Autodesk Inventor part; units mm, degrees
ref_plane "YZ Plane" through (0, 0, 0) normal (1, 0, 0) x (0, 1, 0)
ref_plane "XZ Plane" through (0, 0, 0) normal (0, 1, 0) x (-1, 0, 0)
ref_plane "XY Plane" through (0, 0, 0) normal (0, 0, 1) x (1, 0, 0)
sketch "Sketch1" plane through (0, 0, 0) normal (0, 0, 1) x (1, 0, 0)
  line L0 (-50.8, -25.4) -> (76.2, -25.4)
  line L1 (76.2, -25.4) -> (76.2, 228.6)
  line L2 (76.2, 228.6) -> (-51.6296, 228.6)
  circle A0 centre (5.08, -4.9022) radius 1.905
  circle A1 centre (-1.27, 63.6778) radius 3.175
  circle A2 centre (13.97, 89.0778) radius 3.175
  arc A3 (23.4649, 83.1687) -> (9.3315, 59.465) centre (29.21, 63.6778) ccw
  arc A4 (0.3002, -6.6225) -> (5.08, -9.9822) centre (5.08, -4.9022) ccw
  line L3 (5.08, -9.9822) -> (17.78, -9.9822)
  arc A5 (17.78, -9.9822) -> (22.7496, -3.849) centre (17.78, -4.9022) ccw
  line L4 (9.3315, 59.465) -> (22.7496, -3.849)
  arc A6 (-14.6784, 83.2471) -> (0.3002, -6.6225) centre (239.2924, 79.3933) ccw
  arc A7 (50.546, 191.9478) -> (30.3529, 151.1401) centre (50.546, 166.5478) ccw
  line L5 (50.546, 191.9478) -> (50.546, 210.9978)
  arc A8 (0.9197, 176.5759) -> (0.1225, 170.7438) centre (6.096, 172.8978) ccw
  arc A9 (50.546, 210.9978) -> (0.9197, 176.5759) centre (73.3878, 125.0824) ccw
  arc A10 (-13.9866, 85.1779) -> (0.1225, 170.7438) centre (-83.5064, 140.5873) ccw
  arc A11 (-13.9866, 85.1779) -> (-14.6784, 83.2471) centre (-11.5038, 83.199) ccw
  circle A12 centre (17.78, -4.9022) radius 1.905
  arc A13 (76.2, 171.1429) -> (75.486, 171.3598) centre (64.77, 134.7978) ccw
  arc A14 (30.3529, 151.1401) -> (52.1919, 98.8339) centre (64.77, 134.7978) ccw
  line L6 (-51.6296, 228.6) -> (-51.6296, 223.5757)
  line L7 (-50.8, -9.9822) -> (-50.8, -25.4)
  line L8 (45.5539, 209.5127) -> (50.546, 210.9978)
  arc A15 (55.9788, 92.7525) -> (55.982, 92.7794) centre (50.3052, 93.4393) ccw
  line L9 (48.0499, 210.2553) -> (50.546, 210.9978)
  line L10 (49.298, 210.6265) -> (50.546, 191.9478)
  line L11 (49.298, 210.6265) -> (49.1762, 210.5903)
  line L12 (49.1762, 210.5903) -> (50.546, 191.9478)
  arc A16 (51.9893, 91.5765) -> (52.1919, 98.8339) centre (50.9341, 95.2375) ccw
  line L13 (45.9382, 89.7529) -> (52.0334, 91.5895)
  line L14 (52.0334, 91.5895) -> (23.4649, 83.1687)
  circle A17 centre (13.97, 114.4778) radius 1.905
  circle A18 centre (13.97, 175.4378) radius 1.905
  circle A19 centre (44.6762, 202.1078) radius 1.905
  circle A20 centre (37.7491, 198.9328) radius 1.905
  circle A21 centre (-1.27, 38.2778) radius 1.905
  point P0 (0, 0)
  point P1 (50.546, 87.6896)
  dimension "d1" = 76.2
  dimension "d2" = 25.4
  dimension "d3" = 228.6
  dimension "d5" = 20.4978
  dimension "d6" = 3.81
  dimension "d7" = 6.35
  dimension "d8" = 89.0778
  dimension "d10" = 6.35
  dimension "d11" = 25.4
  dimension "d12" = 15.24
  dimension "d13" = 30.48
  dimension "d14" = 0
  dimension "d15" = 71.12
  dimension "d16" = 35.56
  dimension "d18" = 40.64
  dimension "d22" = 10.16
  dimension "d23" = 12.7
  dimension "d24" = 10.16
  dimension "d28" = 254
  dimension "d29" = 50.8
  dimension "d30" = 14.224
  dimension "d31" = 31.75
  dimension "d33" = 12.7
  dimension "d34" = 44.45
  dimension "d35" = 38.1
  dimension "d36" = 88.9
  dimension "d37" = 88.9
  dimension "d38" = 3.175
  dimension "d39" = 3.81
  dimension "d43" = 5.08
  dimension "d49" = 11.43
  dimension "d50" = 0.127
  dimension "d53" = 1.27
  dimension "d54" = 19.05
  dimension "d55" = 7.62
  dimension "d56" = 3.81
  dimension "d57" = 25.4
  dimension "d58" = 3.81
  dimension "d59" = 60.96
  dimension "d62" = 3.81
  dimension "d63" = 3.81
  dimension "d64" = 7.62
  dimension "d65" = 10.16
  dimension "d66" = 6.985
  dimension "d67" = 3.81
  dimension "d68" = 25.4
extrude "Extrusion6" add sketch "Sketch1" along normal blind 6.35 contours A3 L4 A5 L3 A4 A6 A11 A10 A8 A9 L8 L12 A7 A14 A16 L14 | L12 L8 L10
properties part number "One piece claw 1.0"
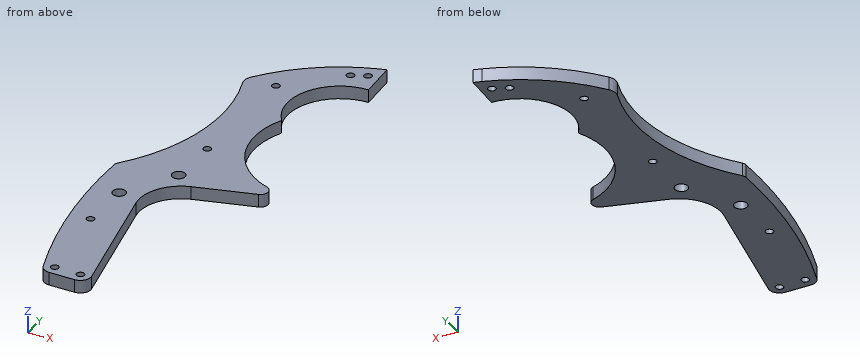
Can you work these out from the model? Positions are in its coordinate system, mm. Give positions to 0.01 mm unless a question says otherwise; leave off trailing zeros. Loops run counter-clockwise (first coordinate to the right, second up) from the corner with the lowest first, then second, coordinate; pieces in that order, holes last. Notation, with made-up numbers: M 39,-1 L 57,-1 A17 cw 57,4 Z; hole C 60,84.25 d7. An arc over 180 degrees is marked long. One line per item, written item: value.
(1) Will these pins go through, and if not, where does the flat tip stop? pin 1 (6 mm diameter, centred on x = 37.75, y = 198.93, fed in from -Z); pin 2 (1 mm diameter, centred on x = 36.5, z = 1, fed in from +Y); pin 3 (3 mm diameter, centred on x = 44.68, y = 202.11, fed in from +Z); pin 4 (3 mm diameter, centred on y = 98, z = 4, fed in from -X).
Returned:
pin 1: z = 0
pin 2: y = 206.19
pin 3: through
pin 4: x = -6.31
(2) Suppose I cut it at B-B on z = 3.5. Count the separate pieces of the cut face and the enclosed holes in it, plus the area to 3 significant figures.
Returned:
separate pieces: 1
enclosed holes: 9
area: 5,990 mm^2
(3) I need wall thicknesses on line 1 (Y direction, x = 44.5, z = 0.5); line 2 (Y direction, x = 36.5, z = 2); line 3 (Y direction, x = 47, z = 2). Which ranges of each line are inside material? Lowest first, please.
Returned:
line 1: 89.37 to 102.54, 191.22 to 200.21, 204 to 209.16
line 2: 87.01 to 109.26, 187.71 to 197.49, 200.37 to 205.97
line 3: 90.11 to 101.1, 191.7 to 209.94
(4) Suppose I cut it at C-C on y = 47.5. List the corners of the cut face in (x, z) for me, plus the area to 3 significant figures.
Returned:
outline: M -12.7,0 L 11.87,0 L 11.87,6.35 L -12.7,6.35 Z
area: 156 mm^2
(5) Suppose I cut it at A-A on x = 13.97. List the corners of the cut face in (y, z) for me.
Returned:
outline: M -9.98,0 L 37.58,0 L 37.58,6.35 L -9.98,6.35 Z; M 77.12,0 L 85.9,0 L 85.9,6.35 L 77.12,6.35 Z; M 92.25,0 L 112.57,0 L 112.57,6.35 L 92.25,6.35 Z; M 116.38,0 L 173.53,0 L 173.53,6.35 L 116.38,6.35 Z; M 177.34,0 L 191.21,0 L 191.21,6.35 L 177.34,6.35 Z
